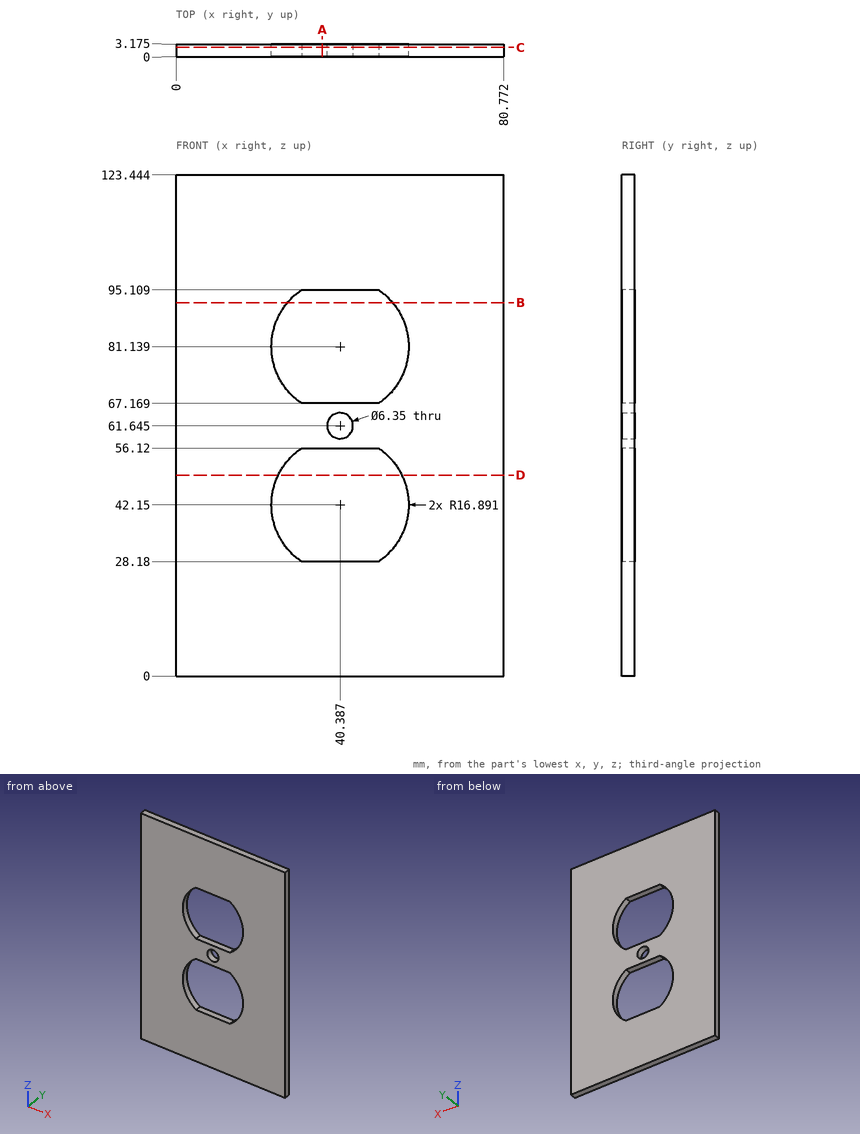
The drawing under review shows one solid part. Ordinate dimensions are in mm from its lowest x, y, z. Give positions to 0.01 mm unless a question says otherwise; leave off trailing zeros. Order: outer loops, then holes, each group sorted by start corner. A loop starts at its lowest first (then second) coordinate and runs counter-clockwise, first axis right, second up. Notation, with made-up numbers: (10, 5.25) - (55, 5.25) arc R31 ccw to (55, 38.25) - close; hole circle Ø6 at (61, 37.25). An arc over 180 degrees is marked (long way). Answer as a JSON object with one key per item and string values. Group by question number.
Item 1: Take a section at B-B on z = 92. Give the boundary of the cut face in (x, y) (1 decimal), and give its area (3 significant figures).
Item 2: Take a section at D-D on z = 49.5. Give the boundary of the cut face in (x, y) (1 decimal).
Item 3: Take a section at C-C on y = 2.35. Give the number of separate pieces and of enclosed holes in the cut face, and give its area (3 significant figures).
Item 4: Clearance check with a flat-ended pin moving along its axis: pin 1 Ø1.5 at (x, y) = (20, 2) entering from -Z. State where the tip first meets the part, or that it passes through.
Item 5: Take a section at A-A on x = 36. Give the boundary of the cut face in (y, z) (1 decimal).
Item 6: Wall thickness on line 1 along Z through (x, y) = (37, 1.85); line 2 along X through (y, z) = (2.95, 42); line 3 along X through (y, z) = (2.05, 29.5) (1 decimal): over which ranges is each line inside the solid? List them lowest first.
Reported:
{
 "1": {"outline": "(0, 0) - (27.5, 0) - (27.5, 3.2) - (0, 3.2) - close; (53.3, 0) - (80.8, 0) - (80.8, 3.2) - (53.3, 3.2) - close", "area": "174 mm^2"},
 "2": {"outline": "(0, 0) - (25.2, 0) - (25.2, 3.2) - (0, 3.2) - close; (55.6, 0) - (80.8, 0) - (80.8, 3.2) - (55.6, 3.2) - close"},
 "3": {"separate pieces": "1", "enclosed holes": "3", "area": "8,300 mm^2"},
 "4": {"pin 1": "z = 0"},
 "5": {"outline": "(0, 0) - (3.2, 0) - (3.2, 28.2) - (0, 28.2) - close; (0, 56.1) - (3.2, 56.1) - (3.2, 67.2) - (0, 67.2) - close; (0, 95.1) - (3.2, 95.1) - (3.2, 123.4) - (0, 123.4) - close"},
 "6": {"line 1": "0 to 28.18, 56.12 to 67.17, 95.11 to 123.44", "line 2": "0 to 23.5, 57.28 to 80.77", "line 3": "0 to 29.2, 51.6 to 80.8"}
}
